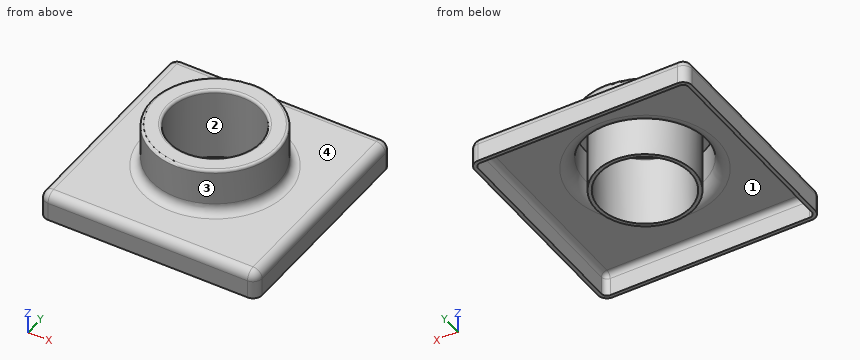
```python
from build123d import *

# Parameters (mm, degrees)
SKETCH2_W           = 120
SKETCH2_H           = 120
BOSS_EXTRUDE1_DEPTH = 15
SKETCH3_R           = 35
BOSS_EXTRUDE2_DEPTH = 25
SKETCH4_R           = 25
CUT_EXTRUDE1_DEPTH  = 175.355957742
FILLET1_R           = 5
FILLET2_R           = 1.5
SHELL1_T            = -2


with BuildPart() as part:
    # Sketch2 → Boss-Extrude1 (new body)
    with BuildSketch(Plane.XY):
        with Locations((60, 60)):
            Rectangle(SKETCH2_W, SKETCH2_H)
    extrude(amount=BOSS_EXTRUDE1_DEPTH)

    # Sketch3 → Boss-Extrude2 (add)
    with BuildSketch(Plane.XY.offset(15)):
        with Locations(Location((60, 60, 0), (0, 0, 180))):
            Circle(SKETCH3_R)
    extrude(amount=BOSS_EXTRUDE2_DEPTH)

    # Sketch4 → Cut-Extrude1 (cut, through all)
    with BuildSketch(Plane.XY.offset(40)):
        with Locations((60, 60)):
            Circle(SKETCH4_R)
    extrude(amount=-CUT_EXTRUDE1_DEPTH, mode=Mode.SUBTRACT)

    # Fillet1
    fillet1_edges = [part.edges().sort_by_distance(p)[0] for p in [
        (120, 60, 15),
        (60, 120, 15),
        (95, 60, 15),
        (0, 60, 15),
        (60, 0, 15),
        (0, 120, 7.5),
        (120, 120, 7.5),
        (120, 0, 7.5),
        (0, 0, 7.5),
    ]]
    fillet(fillet1_edges, radius=FILLET1_R)

    # Fillet2
    fillet2_edges = [part.edges().sort_by_distance(p)[0] for p in [
        (95, 60, 40),
        (35, 60, 40),
    ]]
    fillet(fillet2_edges, radius=FILLET2_R)

    # Shell1
    shell1_openings = [part.faces().sort_by_distance(p)[0] for p in [
        (60, 1.697056275, 0),
    ]]
    offset(amount=SHELL1_T, openings=shell1_openings, kind=Kind.INTERSECTION)


solid = part.part
```
Part model, mm, in its own coordinate system. Face numbers are marked on the shaded views. Give positions to 0.01 mm unless a question says otherwise; leave off trailing zeros. Write each loop counter-clockwise with the first axis right and the second up, starting at its lowest first coordinate (ties: lowest second). Pieces come first, ordered by that corner, then holes. Notation, with made-up numbers: (50.5, 38) -> (63.5, 38) arc R21 ccw to (63.5, 50) -> close; hole circle Ø7 at (23, 21). An arc over 180 degrees is marked (long way). Put each result on its own line as item: value. Start each with the question number.
Item 1: Pull direction Y, two halves, no side cores. Call the marked faces 1, 2, 3 and 4: pulls with the +Y half, pulls with the -Y half, needs draft (parallel to the pull), parting line crosses it, or undercut.
Item 2: Cut at B-B (x = 106). List the corners of the cut face in (y, z), then the cut area to 3 significant figures.
Item 3: Pin check, flat tips, straight feed: pin 1 Ø1.5 at (x, y) = (84, 30) entering from -Z; pin 2 Ø8 at (x, z) = (69, 21) entering from +Y; pin 3 Ø1.5 at (x, z) = (31, 26) entering from -Y. Stop position of each tip, or through.
Item 4: Cut at D-D (z = 17). List the corners of the cut face in (x, y).
Item 5: Wall check: L1, parallel to X at y = 60.5, z = 37 (3 decimals); L2, parallel to Y at x = 60, z = 27.75; L3, parallel to X at y = 9, z = 9.5. Give the ranges that are in metal, low to high. Write a range as [from, to].
Item 6: Cut at A-A (z = 8). List the corners of the cut face in (x, y), then the cut area to 3 significant figures.
Answer list:
1. face 1: undercut
1. face 2: undercut
1. face 3: parting line crosses it
1. face 4: needs draft
2. outline: (0, 0) -> (2, 0) -> (2, 10) arc R3 cw to (5, 13) -> (115, 13) arc R3 cw to (118, 10) -> (118, 0) -> (120, 0) -> (120, 10) arc R5 ccw to (115, 15) -> (5, 15) arc R5 ccw to (0, 10) -> close
2. area: 285 mm2
3. pin 1: stops at z = 13.05
3. pin 2: stops at y = 95.01
3. pin 3: stops at y = 39.34
4. outline: circle Ø72 at (60, 60); circle Ø54 at (60, 60); hole circle Ø67.35 at (60, 60); hole circle Ø50 at (60, 60)
5. L1: x = [25.004, 27.004], [33.005, 35.005], [84.995, 86.995], [92.996, 94.996]
5. L2: y = [25, 27], [33, 35], [85, 87], [93, 95]
5. L3: x = [0, 2], [118, 120]
6. outline: (0, 5) arc R5 ccw to (5, 0) -> (115, 0) arc R5 ccw to (120, 5) -> (120, 115) arc R5 ccw to (115, 120) -> (5, 120) arc R5 ccw to (0, 115) -> close; circle Ø54 at (60, 60); hole (2, 5) arc R3 ccw to (5, 2) -> (115, 2) arc R3 ccw to (118, 5) -> (118, 115) arc R3 ccw to (115, 118) -> (5, 118) arc R3 ccw to (2, 115) -> close; hole circle Ø50 at (60, 60)
6. area: 1,260 mm2
